The drawing under review shows one solid part. Ordinate dimensions are in mm from its lowest x, y, z. A direction names the side the tool comes from. Coordinates: 2 decimals unless noted, no trailing zeros. Loops run counter-clockwise (first coordinate to the right, second up) from the corner with the lowest first, then second, coordinate; pieces in that order, holes last. Notation, with made-up numbers: M 31.25,81.25 L 89.25,81.25 A12 ccw 89.25,96.25 Z; hole C -33.5,14 d10. An arc over 180 degrees is marked long. Return JSON: item names as keys, results as strings.
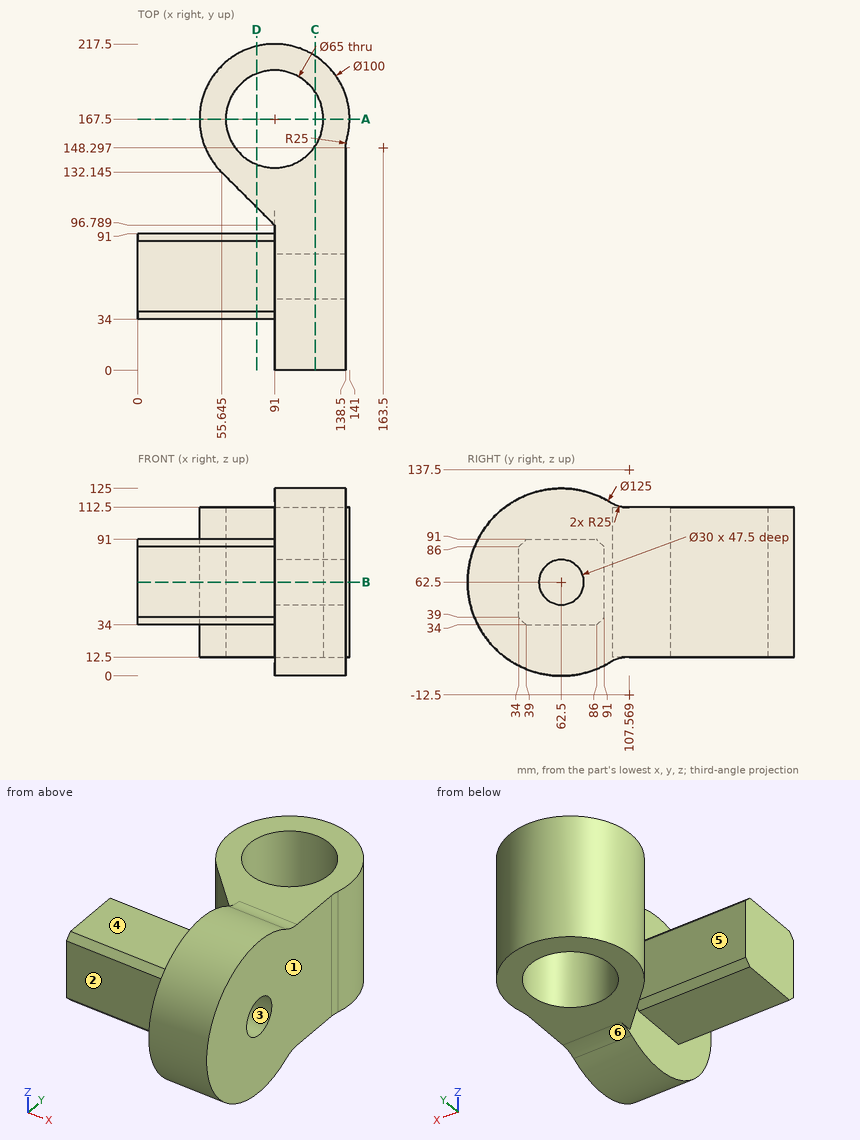
1. Insertion check: pin 1 Ø1.5 at (x, z) = (106.5, 100.5) entering from -Y; pin 2 Ø8 at (y, z) = (70.5, 97) entering from +X; pin 3 Ø5 at (x, z) = (61.5, 76) entering from +Y. Each pin has a flat end and moves straight along its axis. Give the tip position at first contact, or say it passes through.
Check values:
{"pin 1": "y = 12.31", "pin 2": "x = 138.5", "pin 3": "y = 209.58"}
2. Add section C-C on x = 118. Give the boundary of the cut face in (y, z), plus the area to 3 significant figures.
Check values:
{"outline": "M 94.69,8.93 A25 cw 107.57,12.5 L 149.41,12.5 L 149.41,112.5 L 107.57,112.5 A25 cw 94.69,116.07 A62.5 ccw long Z; M 185.59,12.5 L 209.58,12.5 L 209.58,112.5 L 185.59,112.5 Z; hole C 62.5,62.5 d30", "area": "17,200 mm²"}
3. Add section A-A on y = 167.5. Give the boundary of the cut face in (x, z).
Check values:
{"outline": "M 41,12.5 L 58.5,12.5 L 58.5,112.5 L 41,112.5 Z; M 123.5,12.5 L 141,12.5 L 141,112.5 L 123.5,112.5 Z"}
4. Add section D-D on x = 79. Give the boundary of the cut face in (y, z).
Check values:
{"outline": "M 34,39 L 39,34 L 86,34 L 91,39 L 91,86 L 86,91 L 39,91 L 34,86 Z; M 108.79,12.5 L 137.3,12.5 L 137.3,112.5 L 108.79,112.5 Z; M 197.7,12.5 L 216.04,12.5 L 216.04,112.5 L 197.7,112.5 Z"}
5. Machinability: for the marked faces 1, 2 and 3, which of the approach directions +Z, -Z, +X, -X, +Y, -Y give a long, thin tool a straight path to every point of the face, cutting with its end or side? Answer none if there is none.
Check values:
{"face 1": "+Z, -Z, +X, -Y", "face 2": "+Z, -Z, -X, -Y", "face 3": "+X"}
6. Add section B-B on z = 62.5. Give the boundary of the cut face in (x, y) (1 decimal).
Check values:
{"outline": "M 0,34 L 91,34 L 91,0 L 138.5,0 L 138.5,47.5 L 91,47.5 L 91,77.5 L 138.5,77.5 L 138.5,148.3 A25 cw 139.3,154.7 A50 ccw long 55.6,132.1 L 91,96.8 L 91,91 L 0,91 Z; hole C 91,167.5 d65"}
7. To check wall thickness, follow line 1 (X direction, y = 166, z = 97.5) (1 decimal); line 2 (X direction, y = 77, z = 101.5); line 3 (Y direction, x = 76, z = 19) (1 decimal). State the ranges of each line that lie inside material, in increasing order.
Check values:
{"line 1": "41 to 58.5, 123.5 to 141", "line 2": "91 to 138.5", "line 3": "111.8 to 138.7, 196.3 to 215.2"}
8. The part is to be moulded in two halves that separate along Y. For the marked faces 4, 5 and 6, say which applies: released by +Y, released by -Y, zero draft, split by the parting line, or undercut.
Check values:
{"face 4": "zero draft", "face 5": "undercut", "face 6": "released by +Y"}
